from build123d import *

# Parameters (mm, degrees)
F1_DEPTH = 450.85
F2_R     = 5.08
F4_DEPTH = 76.201
F5_R     = 3.17499
F6_R     = 1.397


# Not quite as in the source:
# - a fillet or chamfer is up to 0.001 mm smaller than in the source, because OpenCascade refuses the exact size


with BuildPart() as f1:
    # F0 (on Front) → F1 (new body, symmetric)
    with BuildSketch(Plane.XZ):
        Polygon((76.2, 0), (0, 0), (0, -76.2), (6.35, -76.2), (6.35, -6.35), (76.2, -6.35), align=None)
    extrude(amount=F1_DEPTH, both=True)

    # F2
    f2_edges = [f1.edges().sort_by_distance(p)[0] for p in [
        (6.35, 0, -6.35),
    ]]
    fillet(f2_edges, radius=F2_R)

    # F3 (on Top) → F4 (cut, through all)
    with BuildSketch(Plane.XY):
        Polygon((76.2, 381), (76.2, 450.85), (6.35, 450.85), align=None)
        Polygon((76.2, -450.85), (76.2, -381), (6.35, -450.85), align=None)
    extrude(amount=-F4_DEPTH, mode=Mode.SUBTRACT)

    # F5 (radius 3.175 in the source; OpenCascade refuses exactly that, so slightly less here)
    f5_edges = [f1.edges().sort_by_distance(p)[0] for p in [
        (76.2, 0, -6.35),
        (76.2, 0, 0),
        (0, 0, -76.2),
        (6.35, 0, -76.2),
    ]]
    fillet(f5_edges, radius=F5_R)

    # F6
    f6_edges = [f1.edges().sort_by_distance(p)[0] for p in [
        (0, 0, 0),
    ]]
    fillet(f6_edges, radius=F6_R)


solid = f1.part
Could you check a few things on this model? Use its own coordinates, in mm. A direction names the side the tool comes from. Round coordinates to 2 decimals unless told otherwise and drop trailing zeros. Loops run counter-clockwise (first coordinate to the right, second up) from the corner with the lowest first, then second, coordinate; pieces in that order, holes last. Notation, with made-up numbers: (9.25, 63.5) - (68.25, 63.5) arc R36 ccw to (68.25, 97.5) - close; hole circle Ø7 at (-12.75, 17.5). An arc over 180 degrees is marked (long way). Write item = value, one per line.
1) On a 3-axis mill with a long thin cutter (end or side, diameter ignored), from which of +Z, -Z, +X, -X, +Y, -Y can I reach the whole of each face in a straight line? I mean faces 1 (the flat face through (41.8, -415.4, -3.1)), 2 (the flat face through (6.35, -6, -43)). Say none if no direction works.
Computed:
face_1 = +Z, -Z, +X, -Y
face_2 = -Z, +X, +Y, -Y
2) Imagine slicing it at B-B (x = 20.5). Please give me the cut outline in (y, z).
Computed:
outline = (-436.7, -6.35) - (436.7, -6.35) - (436.7, 0) - (-436.7, 0) - close
3) Imagine slicing it at C-C (z = -63). Please give me the cut outline in (x, y).
Computed:
outline = (0, -450.85) - (6.35, -450.85) - (6.35, 450.85) - (0, 450.85) - close
4) I'm going to push flat-ended pins straight in: P1, Ø18.5, axis at y = -55, z = -54.5, coming from the +X side; P2, Ø12, axis at x = 40.5, z = -10.5, coming from the -Y side; P3, Ø8, axis at x = 36, y = -17, coming from the -Z side. Where does each tip first touch, or does it pass through?
Computed:
P1 = 6.35
P2 = -421.03
P3 = -6.35
5) I need wall thicknesses on line 1 along X through (y, z) = (414, -20); line 2 along Z through (x, y) = (34, 14); line 3 along Z through (x, y) = (11, -127.5). Which ranges of each line are inside material? Lowest first, please. Write a range as from..to.
Computed:
line_1 = 0..6.35
line_2 = -6.35..0
line_3 = -6.37..0
